from build123d import *

# Parameters (mm, degrees)
SKETCH_1_W          = 40
SKETCH_1_H          = 40
EXTRUDE_1_DEPTH     = 18
SKETCH_2_R          = 15
EXTRUDE_2_DEPTH     = 4
SKETCH_3_R          = 5
EXTRUDE_3_DEPTH     = 1
SKETCH_4_R          = 6
EXTRUDE_4_DEPTH     = 12
SKETCH_5_R          = 5
EXTRUDE_5_DEPTH     = 1
SKETCH_6_R          = 6
EXTRUDE_6_DEPTH     = 12.5
SKETCH_8_R          = 2.5
CUT_EXTRUDE_1_DEPTH = 36
SKETCH_9_R          = 4
CUT_EXTRUDE_2_DEPTH = 10
CUT_EXTRUDE_3_REACH = 55.5
SKETCH_10_R         = 2.5
SKETCH_11_R         = 4
CUT_EXTRUDE_4_DEPTH = 10
CHAMFER_1_SIZE      = 0.5
CHAMFER_2_SIZE      = 0.828
CHAMFER_3_SIZE      = 2


with BuildPart() as part:
    # Эскиз1 → Бобышка-Вытянуть1 (new body)
    with BuildSketch(Plane.XY):
        Rectangle(SKETCH_1_W, SKETCH_1_H)
    extrude(amount=EXTRUDE_1_DEPTH)

    # Эскиз2 → Бобышка-Вытянуть2 (add)
    with BuildSketch(Plane.XY.offset(18)):
        Circle(SKETCH_2_R)
    extrude(amount=EXTRUDE_2_DEPTH)

    # Эскиз3 → Бобышка-Вытянуть3 (add)
    with BuildSketch(Plane.XY.offset(22)):
        Circle(SKETCH_3_R)
    extrude(amount=EXTRUDE_3_DEPTH)

    # Эскиз4 → Бобышка-Вытянуть4 (add)
    with BuildSketch(Plane.XY.offset(23)):
        Circle(SKETCH_4_R)
    extrude(amount=EXTRUDE_4_DEPTH)

    # Эскиз5 → Бобышка-Вытянуть5 (add)
    with BuildSketch(Plane.ZY.offset(20)):
        with Locations((7, 0)):
            Circle(SKETCH_5_R)
    extrude(amount=EXTRUDE_5_DEPTH)

    # Эскиз6 → Бобышка-Вытянуть6 (add)
    with BuildSketch(Plane.ZY.offset(21)):
        with Locations((7, 0)):
            Circle(SKETCH_6_R)
    extrude(amount=EXTRUDE_6_DEPTH)

    # Эскиз7 → Вырез-Повернуть1 (revolve, cut)
    with BuildSketch(Plane(origin=(0, 0, 0), x_dir=(1, 0, 0), z_dir=(0, 1, 0))):
        Polygon((0, 0), (0, -8), (3.5, -8), (8.696152423, -11), (11, -11), (11, 0), align=None)
    revolve(axis=Axis((0, 0, 0), (0, 0, 1)), mode=Mode.SUBTRACT)

    # Эскиз8 → Вырез-Вытянуть1 (cut, through all)
    with BuildSketch(Plane.XY.offset(35)):
        Circle(SKETCH_8_R)
    extrude(amount=-CUT_EXTRUDE_1_DEPTH, mode=Mode.SUBTRACT)

    # Эскиз9 → Вырез-Вытянуть2 (cut)
    with BuildSketch(Plane.XY.offset(35)):
        Circle(SKETCH_9_R)
    extrude(amount=-CUT_EXTRUDE_2_DEPTH, mode=Mode.SUBTRACT)

    # Эскиз10 → Вырез-Вытянуть3 (cut, up to next)
    with BuildSketch(Plane.ZY.offset(33.5), mode=Mode.PRIVATE) as cut_extrude_3_sk1:
        with Locations((7, 0)):
            Circle(SKETCH_10_R)
    cut_extrude_3_tool1 = extrude(cut_extrude_3_sk1.sketch, amount=-CUT_EXTRUDE_3_REACH, mode=Mode.PRIVATE) & part.part
    add(cut_extrude_3_tool1.solids().sort_by_distance((-33.5, 0, 7))[0], mode=Mode.SUBTRACT)

    # Эскиз11 → Вырез-Вытянуть4 (cut)
    with BuildSketch(Plane.ZY.offset(33.5)):
        with Locations((7, 0)):
            Circle(SKETCH_11_R)
    extrude(amount=-CUT_EXTRUDE_4_DEPTH, mode=Mode.SUBTRACT)

    # Фаска1
    chamfer_1_edges = [part.edges().sort_by_distance(p)[0] for p in [
        (-4, 0, 35),
        (-33.5, 0, 3),
    ]]
    chamfer(chamfer_1_edges, length=CHAMFER_1_SIZE)

    # Фаска2
    chamfer_2_edges = [part.edges().sort_by_distance(p)[0] for p in [
        (-6, 0, 35),
        (-33.5, 0, 1),
    ]]
    chamfer(chamfer_2_edges, length=CHAMFER_2_SIZE)

    # Фаска3
    chamfer_3_edges = [part.edges().sort_by_distance(p)[0] for p in [
        (20, -20, 9),
        (-20, -20, 9),
        (-20, 20, 9),
        (20, 20, 9),
    ]]
    chamfer(chamfer_3_edges, length=CHAMFER_3_SIZE)

    # Эскиз12 → Вырез-Повернуть2 (revolve, cut)
    with BuildSketch(Plane(origin=(0, 0, 0), x_dir=(1, 0, 0), z_dir=(0, 1, 0))):
        with BuildLine():
            Line((13.5, 0), (13.5, 3))
            ThreePointArc((13.5, 3), (15.5, 5), (17.5, 3))
            Line((17.5, 3), (17.5, 0))
            ThreePointArc((17.5, 0), (15.5, -2), (13.5, 0))
        make_face()
    revolve(axis=Axis((0, 0, 0), (0, 0, 1)), mode=Mode.SUBTRACT)


solid = part.part
Part model, mm, in its own coordinate system. A direction names the side the tool comes from. Round coordinates to 2 decimals unless told otherwise and drop trailing zeros. Write each loop counter-clockwise with the first axis right and the second up, starting at its lowest first coordinate (ties: lowest second). Pieces come first, ordered by that corner, then holes. Notation, with made-up numbers: (89, 19.5) - (133, 19.5) arc R16 cw to (133, 48.5) - close; hole circle Ø6 at (-21, -10). An arc over 180 degrees is marked (long way). Use CSV: the item, a comma, the result in double quotes.
Item 1: Slice it at B-B, the plane z = 7. Write the cut outline in (x, y), then the cut area to 3 significant figures.
Results list:
outline,"(-33.5, -5.17) - (-32.67, -6) - (-21, -6) - (-21, -5) - (-20, -5) - (-20, -18) - (-18, -20) - (18, -20) - (20, -18) - (20, 18) - (18, 20) - (-18, 20) - (-20, 18) - (-20, 5) - (-21, 5) - (-21, 6) - (-32.67, 6) - (-33.5, 5.17) - (-33.5, 4.5) - (-33, 4) - (-23.5, 4) - (-23.5, 2.5) - (-10.71, 2.5) arc R11 cw (long way) to (-10.71, -2.5) - (-23.5, -2.5) - (-23.5, -4) - (-33, -4) - (-33.5, -4.5) - close"
area,"1,230 mm²"
Item 2: Pull direction Y, two halves, no side cores. Call faces 5 (the cylindrical face through (-0.867, -3.905, 29.816)), 6 (the flat face through (19, -19, 9)), 7 (the flat face through (-4, 4, 22)), 8 (the flat face through (0, 20, 9)): pulls with the +Y half, pulls with the -Y half, needs draft (parallel to the pull), parting line crosses it, or undercut.
Results list:
face 5,"undercut"
face 6,"pulls with the -Y half"
face 7,"needs draft"
face 8,"pulls with the +Y half"
Item 3: Wall check: L1, parallel to Y at x = 0, z = 13; L2, parallel to Y at x = 0, z = 32; L3, parallel to Z at x = -19, y = -9. Give the ranges that are in metal, low to high.
Results list:
L1,"y = -20 to -2.5, 2.5 to 20"
L2,"y = -6 to -4, 4 to 6"
L3,"z = 0 to 18"
Item 4: Slice it at A-A, the plane z = 19. Write the cut outline in (x, y), then the cut area to 3 significant figures.
Results list:
outline,"circle Ø30 at (0, 0); hole circle Ø5 at (0, 0)"
area,"687 mm²"
Item 5: Slice it at C-C, the plane z = 27.5. Write the cut outline in (x, y).
Results list:
outline,"circle Ø12 at (0, 0); hole circle Ø8 at (0, 0)"
Item 6: Flat gauge pins, fed straight in: P1, Ø2, axis at x = -1.5, y = 1, coming from the -Z side; P2, Ø5, axis at y = 8.5, z = 5.5, coming from the -X side; P3, Ø2.5, axis at y = -1, z = 7.5, coming from the -X side. Where does each tip first touch, or does it go through?
Results list:
P1,"stops at z = 8"
P2,"stops at x = -20"
P3,"stops at x = -4.71"
Item 7: Tool access for faces 1 (the cylindrical face through (-1.08, -4.88, 22.49)), 2 (the cylindrical face through (-14.985, 0.66, 19.972)), 3 (the flat face through (-5, -10, 0)), 4 (the cylindrical face through (-28.3, -2.4, 3.8)): list every direction of +Z, -Z, +X, -X, +Y, -Y with a clear straight run to the whole face (end or side of a thin tool).
Results list:
face 1,"none"
face 2,"+Z"
face 3,"-Z, +X, -X, +Y, -Y"
face 4,"-X"
